from build123d import *

# Parameters (mm, degrees)
BOSS_EXTRUDE3_DEPTH             = 2
SKETCH3_R                       = 3
BOSS_EXTRUDE4_DEPTH             = 9
BOSS_EXTRUDE5_DEPTH             = 38.5
BOSS_EXTRUDE5_DEPTH_BACK        = 38.5
SWEEP2_START                    = 11
SWEEP2_DEPTH                    = 78
SWEEP2_2_DEPTH                  = 8
SWEEP2_START_2                  = -4
SWEEP2_3_DEPTH                  = 8
SWEEP4_START                    = 11
SWEEP4_DEPTH                    = 78
SWEEP4_2_DEPTH                  = 8
SWEEP4_START_2                  = -4
SWEEP4_3_DEPTH                  = 8
BOSS_EXTRUDE6_DEPTH             = 3
BOSS_EXTRUDE6_DIRECTION_2_REACH = 128.768
BOSS_EXTRUDE7_DEPTH             = 3
BOSS_EXTRUDE7_DEPTH_BACK        = 3


with BuildPart() as part:
    # Sketch2 → Boss-Extrude3 (new body)
    with BuildSketch(Plane(origin=(0, 0, 0), x_dir=(1, 0, 0), z_dir=(0, 1, 0))):
        with BuildLine():
            add(Edge.make_bspline(
                [(-2.354354779, -2.354354779), (0, -20.812496246), (2.354354779, -2.354354779)],
                knots=[5.055412921, 5.055412921, 5.055412921, 7.510957694, 7.510957694, 7.510957694], degree=2, weights=[1, 0.336336397, 1]))
            add(Edge.make_bspline(
                [(2.354354779, -2.354354779), (20.812496246, 0), (2.354354779, 2.354354779)],
                knots=[1.913820267, 1.913820267, 1.913820267, 4.36936504, 4.36936504, 4.36936504], degree=2, weights=[1, 0.336336397, 1]))
            add(Edge.make_bspline(
                [(2.354354779, 2.354354779), (0, 20.812496246), (-2.354354779, 2.354354779)],
                knots=[1.913820267, 1.913820267, 1.913820267, 4.36936504, 4.36936504, 4.36936504], degree=2, weights=[1, 0.336336397, 1]))
            add(Edge.make_bspline(
                [(-2.354354779, 2.354354779), (-20.812496246, 0), (-2.354354779, -2.354354779)],
                knots=[5.055412921, 5.055412921, 5.055412921, 7.510957694, 7.510957694, 7.510957694], degree=2, weights=[1, 0.336336397, 1]))
        make_face()
    extrude(amount=BOSS_EXTRUDE3_DEPTH)

    # Sketch3 → Boss-Extrude4 (add)
    with BuildSketch(Plane(origin=(0, 2, 0), x_dir=(1, 0, 0), z_dir=(0, 1, 0))):
        with Locations(Location((0, 0, 0), (0, 0, 270))):
            Circle(SKETCH3_R)
    extrude(amount=BOSS_EXTRUDE4_DEPTH)

    # Sketch4 → Boss-Extrude5 (add, two sides: drawn at the far end of the back side and taken through both)
    with BuildSketch(Plane(origin=(0, 0, 0), x_dir=(0, 0, -1), z_dir=(1, 0, 0)).offset(-BOSS_EXTRUDE5_DEPTH_BACK)):
        with BuildLine():
            Line((3, 11), (-3, 11))
            Line((-3, 11), (-3, 14))
            ThreePointArc((-3, 14), (0, 17), (3, 14))
            Line((3, 14), (3, 11))
        make_face()
    extrude(amount=BOSS_EXTRUDE5_DEPTH + BOSS_EXTRUDE5_DEPTH_BACK)



with BuildPart() as body_2:
    # Sweep2: read off the stored shape, not the designer's step
    # Sweep2 outline → Sweep2 (new body)
    with BuildSketch(Plane(origin=(0, 0, 0), x_dir=(1, 0, 0), z_dir=(0, 1, 0)).offset(SWEEP2_START)):
        with BuildLine():
            Line((46.5, -3), (46.5, 3))
            Line((46.5, 3), (43.5, 3))
            ThreePointArc((43.5, 3), (40.5, 0), (43.5, -3))
            Line((43.5, -3), (46.5, -3))
        make_face()
    extrude(amount=SWEEP2_DEPTH)


with BuildPart() as part_1:
    add(part.part)

    add(body_2.part)  # Sweep2 2 merges body 2
    # Sweep2 2 outline → Sweep2 2 (add)
    with BuildSketch(Plane(origin=(0, 0, 0), x_dir=(1, 0, 0), z_dir=(0, 1, 0)).offset(SWEEP2_START)):
        with BuildLine():
            ThreePointArc((43.5, -3), (40.5, 0), (43.5, 3))
            Line((43.5, 3), (38.5, 3))
            Line((38.5, 3), (38.5, -3))
            Line((38.5, -3), (43.5, -3))
        make_face()
    extrude(amount=SWEEP2_2_DEPTH)

    # Sweep2 3 outline → Sweep2 3 (cut)
    with BuildSketch(Plane.XY.offset(SWEEP2_START_2)):
        with BuildLine():
            ThreePointArc((46.5, 19), (44.156854249, 13.343145751), (38.5, 11))
            Line((38.5, 11), (46.5, 11))
            Line((46.5, 11), (46.5, 19))
        make_face()
    extrude(amount=SWEEP2_3_DEPTH, mode=Mode.SUBTRACT)

    # Sweep2 4 outline → Sweep2 4 (revolve, cut)
    with BuildSketch(Plane(origin=(38.5, 19, 0), x_dir=(1, 0, 0), z_dir=(0, -1, 0))):
        with BuildLine():
            ThreePointArc((5, -3), (2, 0), (5, 3))
            Line((5, 3), (0, 3))
            Line((0, 3), (0, -3))
            Line((0, -3), (5, -3))
        make_face()
    revolve(axis=Axis((38.5, 19, 0), (0, 0, 1)), mode=Mode.SUBTRACT)



with BuildPart() as body_2_2:
    # Sweep4: read off the stored shape, not the designer's step
    # Sweep4 outline → Sweep4 (new body)
    with BuildSketch(Plane(origin=(0, 0, 0), x_dir=(1, 0, 0), z_dir=(0, 1, 0)).offset(SWEEP4_START)):
        with BuildLine():
            ThreePointArc((-43.5, -3), (-40.5, 0), (-43.5, 3))
            Line((-43.5, 3), (-46.5, 3))
            Line((-46.5, 3), (-46.5, -3))
            Line((-46.5, -3), (-43.5, -3))
        make_face()
    extrude(amount=SWEEP4_DEPTH)


with BuildPart() as part_2:
    add(part_1.part)

    add(body_2_2.part)  # Sweep4 2 merges body 2 2
    # Sweep4 2 outline → Sweep4 2 (add)
    with BuildSketch(Plane(origin=(0, 0, 0), x_dir=(1, 0, 0), z_dir=(0, 1, 0)).offset(SWEEP4_START)):
        with BuildLine():
            Line((-38.5, -3), (-38.5, 3))
            Line((-38.5, 3), (-43.5, 3))
            ThreePointArc((-43.5, 3), (-40.5, 0), (-43.5, -3))
            Line((-43.5, -3), (-38.5, -3))
        make_face()
    extrude(amount=SWEEP4_2_DEPTH)

    # Sweep4 3 outline → Sweep4 3 (cut)
    with BuildSketch(Plane.XY.offset(SWEEP4_START_2)):
        with BuildLine():
            Line((-46.5, 11), (-38.5, 11))
            ThreePointArc((-38.5, 11), (-44.156854249, 13.343145751), (-46.5, 19))
            Line((-46.5, 19), (-46.5, 11))
        make_face()
    extrude(amount=SWEEP4_3_DEPTH, mode=Mode.SUBTRACT)

    # Sweep4 4 outline → Sweep4 4 (revolve, cut)
    with BuildSketch(Plane(origin=(-38.5, 19, 0), x_dir=(1, 0, 0), z_dir=(0, -1, 0))):
        with BuildLine():
            Line((0, -3), (5, -3))
            ThreePointArc((5, -3), (2, 0), (5, 3))
            Line((5, 3), (0, 3))
            Line((0, 3), (0, -3))
        make_face()
    revolve(axis=Axis((-38.5, 19, 0), (0, 0, 1)), mode=Mode.SUBTRACT)

    # Sketch8 → Boss-Extrude6 (add)
    with BuildSketch(Plane(origin=(-43.5, 0, 0), x_dir=(0, 0, -1), z_dir=(1, 0, 0))):
        with BuildLine():
            Line((20.5, 109), (18, 109))
            ThreePointArc((18, 109), (0, 91), (-18, 109))
            Line((-18, 109), (-20.5, 109))
            ThreePointArc((-20.5, 109), (0, 88.5), (20.5, 109))
        make_face()
    extrude(amount=BOSS_EXTRUDE6_DEPTH)

    # Boss-Extrude6 direction 2: up to this face of the body (flat: up to its plane)
    boss_extrude6_direction_2_end = Plane(part_2.part.faces().sort_by_distance((-46.5, 54, 0))[0])
    # Sketch8 → Boss-Extrude6 direction 2 (add, up to the picked face)
    with BuildSketch(Plane(origin=(-43.5, 0, 0), x_dir=(0, 0, -1), z_dir=(1, 0, 0)), mode=Mode.PRIVATE) as boss_extrude6_direction_2_sk1:
        with BuildLine():
            Line((20.5, 109), (18, 109))
            ThreePointArc((18, 109), (0, 91), (-18, 109))
            Line((-18, 109), (-20.5, 109))
            ThreePointArc((-20.5, 109), (0, 88.5), (20.5, 109))
        make_face()
    boss_extrude6_direction_2_tool1 = split(extrude(boss_extrude6_direction_2_sk1.sketch, amount=-BOSS_EXTRUDE6_DIRECTION_2_REACH, mode=Mode.PRIVATE), bisect_by=boss_extrude6_direction_2_end, keep=Keep.BOTH, mode=Mode.PRIVATE)
    add(boss_extrude6_direction_2_tool1.solids().sort_by(Axis((-43.5, 108.541606, -19.25), (-1, 0, 0)))[0])

    # Sketch9 → Boss-Extrude7 (add, two sides: drawn at the far end of the back side and taken through both)
    with BuildSketch(Plane(origin=(43.5, 0, 0), x_dir=(0, 0, -1), z_dir=(1, 0, 0)).offset(-BOSS_EXTRUDE7_DEPTH_BACK)):
        with BuildLine():
            Line((-18, 109), (-20.5, 109))
            ThreePointArc((-20.5, 109), (0, 88.5), (20.5, 109))
            Line((20.5, 109), (18, 109))
            ThreePointArc((18, 109), (0, 91), (-18, 109))
        make_face()
    extrude(amount=BOSS_EXTRUDE7_DEPTH + BOSS_EXTRUDE7_DEPTH_BACK)


solid = part_2.part
Verification items for the finished model (mm, model axes). A direction names the side the tool comes from. Coordinates: 2 decimals unless noted, no trailing zeros. Order: outer loops, then holes, each group sorted by start corner. A loop starts at its lowest first (then second) coordinate and runs counter-clockwise, first axis right, second up. Notation, with made-up numbers: M 79.25,23 L 119.25,23 A12 ccw 119.25,29 Z; hole C 89.25,-36.5 d6. An arc over 180 degrees is marked long. Return JSON: item names as keys, results as strings.
1) Cross-section at C-C, the plane y = 95. Record the boundary of the cut face in (x, z), and give its area (3 significant figures).
Answer list:
{"outline": "M -46.5,-14.97 L -40.5,-14.97 L -40.5,-11.31 L -46.5,-11.31 Z; M -46.5,11.31 L -40.5,11.31 L -40.5,14.97 L -46.5,14.97 Z; M 40.5,-14.97 L 46.5,-14.97 L 46.5,-11.31 L 40.5,-11.31 Z; M 40.5,11.31 L 46.5,11.31 L 46.5,14.97 L 40.5,14.97 Z", "area": "87.9 mm2"}
2) Cross-section at A-A, the plane y = 60. Record the boundary of the cut face in (x, z).
Answer list:
{"outline": "M -46.5,-3 L -43.5,-3 A3 ccw -43.5,3 L -46.5,3 Z; M 43.5,-3 L 46.5,-3 L 46.5,3 L 43.5,3 A3 ccw Z"}
3) Cross-section at B-B, the plane z = -10.5. Record the boundary of the cut face in (x, y), and give its area (3 significant figures).
Answer list:
{"outline": "M -46.5,91.39 L -40.5,91.39 L -40.5,94.38 L -46.5,94.38 Z; M 40.5,91.39 L 46.5,91.39 L 46.5,94.38 L 40.5,94.38 Z", "area": "35.8 mm2"}
4) Thickness scan on L1, parallel to X at y = 92, z = -11; L2, parallel to X at y = 77, z = 1; L3, parallel to Z at x = -18.5, y = 13. Record the ranges inside material, lowest first. Write a range as [from, to].
Answer list:
{"L1": "[-46.5, -40.5], [40.5, 46.5]", "L2": "[-46.5, -40.67], [40.67, 46.5]", "L3": "[-3, 3]"}
5) Cross-section at D-D, the plane x = 33. Record the boundary of the cut face in (y, z), and give its area (3 significant figures).
Answer list:
{"outline": "M 11,-3 L 14,-3 A3 ccw 14,3 L 11,3 Z", "area": "32.1 mm2"}
6) Access from +Z, -Z, +X, -X, +Y, -Y to the whole of each face (thin tool, end or side, straight path). Record for faces 1 (the cylindrical face through (-40.5, 53.4, 0.1)), 2 (the cylindrical face through (43, 91, 0)).
Answer list:
{"face 1": "none", "face 2": "+X, -X, +Y"}
7) Gauge pin test, flat ends, axial feed: pin 1 (5 mm diameter, centred on x = 10, z = 1, fed in from -Y); pin 2 (4 mm diameter, centred on x = -1.5, z = -2, fed in from +Y); pin 3 (16.5 mm diameter, centred on y = 102.5, z = 3.5, fed in from +X). Record the tip position at first contact, or that the pin passes through.
Answer list:
{"pin 1": "y = 11", "pin 2": "y = 17", "pin 3": "through"}
8) Release check for a two-part mould opening along X. For faces 3 (the flat face through (43, 109, 19)), 4 (the cylindrical face through (-1, 17, 0)), 5 (the cylindrical face through (44.219, 13.406, -0.042)) record: +X half, -X half, draft (parallel to the pull), parting line (faces both ways), or undercut.
Answer list:
{"face 3": "draft", "face 4": "undercut", "face 5": "+X half"}
